from build123d import *

# Parameters (mm, degrees)
ESQUISSE1_W             = 90
ESQUISSE1_H             = 30
BOSS_EXTRU_1_DEPTH      = 23
ESQUISSE2_W             = 13.2
ESQUISSE2_H             = 13.2
ESQUISSE2_W_2           = 2
ESQUISSE2_H_2           = 5
ENL_V_MAT_EXTRU_1_DEPTH = 31
ESQUISSE3_R             = 4
ENL_V_MAT_EXTRU_2_DEPTH = 24
ENL_V_MAT_EXTRU_3_DEPTH = 24
CONG_1_R                = 1


with BuildPart() as part:
    # Esquisse1 → Boss.-Extru.1 (new body)
    with BuildSketch(Plane.XY):
        with Locations((40.889968792, -13.091136671)):
            Rectangle(ESQUISSE1_W, ESQUISSE1_H)
    extrude(amount=BOSS_EXTRU_1_DEPTH)

    # Esquisse2 → Enlèv. mat.-Extru.1 (cut, through all)
    with BuildSketch(Plane(origin=(0, 1.908863329, 0), x_dir=(1, 0, 0), z_dir=(0, 1, 0))):
        with Locations((40.889968792, -11.5)):
            Rectangle(ESQUISSE2_W, ESQUISSE2_H)
        with Locations((48.489968792, -11.5)):
            Rectangle(ESQUISSE2_W_2, ESQUISSE2_H_2)
    extrude(amount=-ENL_V_MAT_EXTRU_1_DEPTH, mode=Mode.SUBTRACT)

    # Esquisse3 → Enlèv. mat.-Extru.2 (cut, through all)
    with BuildSketch(Plane(origin=(0, 0, 0), x_dir=(-1, 0, 0), z_dir=(0, 0, -1))):
        with Locations((-10.889968792, -13.091136671)):
            Circle(ESQUISSE3_R)
        with Locations((-70.889968792, -13.091136671)):
            Circle(ESQUISSE3_R)
    extrude(amount=-ENL_V_MAT_EXTRU_2_DEPTH, mode=Mode.SUBTRACT)

    # Esquisse4 → Enlèv. mat.-Extru.3 (cut, through all)
    with BuildSketch(Plane(origin=(0, 0, 0), x_dir=(-1, 0, 0), z_dir=(0, 0, -1))):
        with BuildLine():
            ThreePointArc((-38.189968792, -8.091136671), (-40.889968792, -10.791136671), (-43.589968792, -8.091136671))
            Line((-43.589968792, -8.091136671), (-43.589968792, -3.091136671))
            ThreePointArc((-43.589968792, -3.091136671), (-40.889968792, -0.391136671), (-38.189968792, -3.091136671))
            Line((-38.189968792, -3.091136671), (-38.189968792, -8.091136671))
        make_face()
        with BuildLine():
            Line((-43.589968792, -23.091136671), (-43.589968792, -18.091136671))
            ThreePointArc((-43.589968792, -18.091136671), (-40.889968792, -15.391136671), (-38.189968792, -18.091136671))
            Line((-38.189968792, -18.091136671), (-38.189968792, -23.091136671))
            ThreePointArc((-38.189968792, -23.091136671), (-40.889968792, -25.791136671), (-43.589968792, -23.091136671))
        make_face()
    extrude(amount=-ENL_V_MAT_EXTRU_3_DEPTH, mode=Mode.SUBTRACT)

    # Congé1
    cong_1_edges = [part.edges().sort_by_distance(p)[0] for p in [
        (47.489968792, -13.091136671, 9),
        (47.489968792, -13.091136671, 14),
    ]]
    fillet(cong_1_edges, radius=CONG_1_R)


solid = part.part
Design review of the part built by this model. Coordinates are the model's own, in mm. A direction names the side the tool comes from. Coordinates: 2 decimals unless noted, no trailing zeros. Write each loop counter-clockwise with the first axis right and the second up, starting at its lowest first coordinate (ties: lowest second). Pieces come first, ordered by that corner, then holes. Notation, with made-up numbers: (-40, -34.5) -> (17, -34.5) arc R15 cw to (17, -17.5) -> close; hole circle Ø7 at (39, 28.5). An arc over 180 degrees is marked (long way). Write each question's results on one line, items separated by ' | '. Start each with the question number.
(1) Tool access review of faces 1 (the face through (85.89, -13, 11)), 2 (the face through (40.95, -15.39, 20.52)), 3 (the face through (41, -13, 18.1)): name each direction out of +Z, -Z, +X, -X, +Y, -Y from which nothing blocks a thin tool from reaching the whole face with its end or side.
(2) The part is to be moulded in two halves that separate along X. For faces 4 (the face through (-4.11, -13, 11)), 5 (the face through (40.83, -25.79, 2.42)), 6 (the face through (40, -13, 0)), say which applies: pulls with the +X half, pulls with the -X half, needs draft (parallel to the pull), parting line crosses it, or undercut.
(3) Take a section at C-C on y = -14.25. Write out the cut boundary in (x, z).
(4) Take a section at B-B on y = -5.25. Write out the cut boundary in (x, z), and give its area (3 significant figures).
(5) Take a section at D-D on z = 20.5. Write out the cut boundary in (x, y), and give its area (3 significant figures).
(6) Take a section at A-A on x = 35.5. Write out the cut boundary in (y, z), and give its area (3 significant figures).
(7) For line 1 along X through (y, z) = (-19.5, 12.25); line 2 along X through (y, z) = (-7.5, 4.25); line 3 along X through (y, z) = (-14.5, 13.5), list the stretches that pass through material, from the lowest coordinate up. Write a range as from..to.
Results found:
1) face 1: +Z, -Z, +X, +Y, -Y | face 2: +Z, -Z | face 3: +Y, -Y
2) face 4: pulls with the -X half | face 5: undercut | face 6: needs draft
3) outline: (-4.11, 0) -> (7.06, 0) -> (7.06, 23) -> (-4.11, 23) -> close; (14.72, 0) -> (67.06, 0) -> (67.06, 23) -> (14.72, 23) -> close; (74.72, 0) -> (85.89, 0) -> (85.89, 23) -> (74.72, 23) -> close; hole (34.29, 4.9) -> (47.49, 4.9) -> (47.49, 8) arc R1 cw to (48.49, 9) -> (49.49, 9) -> (49.49, 14) -> (48.49, 14) arc R1 cw to (47.49, 15) -> (47.49, 18.1) -> (34.29, 18.1) -> close
4) outline: (-4.11, 0) -> (38.19, 0) -> (38.19, 4.9) -> (34.29, 4.9) -> (34.29, 18.1) -> (38.19, 18.1) -> (38.19, 23) -> (-4.11, 23) -> close; (43.59, 0) -> (85.89, 0) -> (85.89, 23) -> (43.59, 23) -> (43.59, 18.1) -> (47.49, 18.1) -> (47.49, 15) arc R1 ccw to (48.49, 14) -> (49.49, 14) -> (49.49, 9) -> (48.49, 9) arc R1 ccw to (47.49, 8) -> (47.49, 4.9) -> (43.59, 4.9) -> close | area: 1,830 mm2
5) outline: (-4.11, -28.09) -> (85.89, -28.09) -> (85.89, 1.91) -> (-4.11, 1.91) -> close; hole circle Ø8 at (10.89, -13.09); hole (38.19, -23.09) arc R2.7 ccw to (43.59, -23.09) -> (43.59, -18.09) arc R2.7 ccw to (38.19, -18.09) -> close; hole (38.19, -8.09) arc R2.7 ccw to (43.59, -8.09) -> (43.59, -3.09) arc R2.7 ccw to (38.19, -3.09) -> close; hole circle Ø8 at (70.89, -13.09) | area: 2,500 mm2
6) outline: (-28.09, 0) -> (1.91, 0) -> (1.91, 4.9) -> (-28.09, 4.9) -> close; (-28.09, 18.1) -> (1.91, 18.1) -> (1.91, 23) -> (-28.09, 23) -> close | area: 294 mm2
7) line 1: x = -4.11..34.29, 49.49..85.89 | line 2: x = -4.11..38.19, 43.59..85.89 | line 3: x = -4.11..7.15, 14.63..34.29, 49.49..67.15, 74.63..85.89
